Autodesk Inventor part; units mm, degrees
ref_plane "YZ Plane" through (0, 0, 0) normal (1, 0, 0) x (0, 1, 0)
ref_plane "XZ Plane" through (0, 0, 0) normal (0, 1, 0) x (-1, 0, 0)
ref_plane "XY Plane" through (0, 0, 0) normal (0, 0, 1) x (1, 0, 0)
sketch "Original Profile" plane through (0, 0, 0) normal (0, 1, 0) x (-1, 0, 0)
  line L0 (0, 0) -> (-18, 0)
  line L1 (-18, 0) -> (-18, -15)
  line L2 (-18, -15) -> (0, -15)
  line L3 (0, -15) -> (0, 0)
  line L4 (0, -7.5) -> (-18, -7.5)
  circle A0 centre (-11.5, -7.5) radius 1.5
  circle A1 centre (-11.5, -7.5) radius 6.5
  line L5 (-5, -15) -> (-5, 0)
  line L6 (0, -9.0875) -> (-18, -9.0875)
  line L7 (-18, -9.0875) -> (-18, -5.9125)
  line L8 (-18, -5.9125) -> (0, -5.9125)
  line L9 (0, -5.9125) -> (0, -9.0875)
  point P0 (0, -5.9125)
  point P1 (-18, -9.0875)
  dimension "d8" = 3
  dimension "d9" = 13
  dimension "d10" = 15
  dimension "d11" = 11.5
  dimension "d12" = 6.5
  dimension "d15" = 5
  dimension "d32" = 3.175
  dimension "d33" = 3.175
extrude "Stock" add sketch "Original Profile" along normal blind 29.25
sketch "Sketch4" plane through (18, 0, 0) normal (1, 0, 0) x (0, 0, -1)
  line L0 (15, 0) -> (15, 29.25)
  line L1 (0, 21.75) -> (15, 21.75)
  line L2 (15, 21.75) -> (15, 3.75)
  line L3 (15, 3.75) -> (0, 3.75)
  line L4 (0, 3.75) -> (0, 21.75)
  line L5 (0, 0) -> (0, 29.25)
  line L6 (0, 0) -> (15, 0)
  line L7 (15, 29.25) -> (0, 29.25)
  line L8 (7.5, 29.25) -> (7.5, 0) construction
  line L9 (15, 0) -> (0, 0)
  line L10 (2.7375, 0) -> (12.2625, 0)
  line L11 (12.2625, 0) -> (12.2625, 1.5)
  line L12 (12.2625, 1.5) -> (2.7375, 1.5)
  line L13 (2.7375, 1.5) -> (2.7375, 0)
  line L14 (2.7375, 1.5) -> (3.6035, 0)
  line L15 (2.7375, 1.5) -> (4.4696, 1.5) construction
  line L16 (12.2625, 1.5) -> (11.3965, 0)
  line L17 (12.2625, 1.5) -> (13.9946, 1.5) construction
  dimension "d40" = 3.75
  dimension "d41" = 18
  dimension "d44" = 9.525
  dimension "d45" = 4.7625
  dimension "d46" = 1.5
  dimension "d47" = 60
  dimension "d48" = 120
extrude "Cut Slot" cut sketch "Sketch4" against normal blind 14 contours L3 L4 L1 L0
extrude "Extrusion7" cut sketch "Sketch4" against normal through all contours L6 L14 L12 L16
hole "Hole1" at (11.5, 0, -7.5) direction (0, 1, 0) diameter 3.2004 end through all
sketch "Sketch5" plane through (0, 0, 0) normal (-1, 0, 0) x (0, 0, 1)
  circle A0 centre (-7.5, 14.625) radius 1.5
  line L0 (-15, 29.25) -> (0, 29.25)
  line L1 (-15, 0) -> (-11.3965, 0)
  line L2 (-15, 0) -> (-15, 29.25)
  point P0 (0, 0)
  dimension "d51" = 3
  dimension "d52" = 14.625
  dimension "d53" = 29.25
  dimension "d54" = 7.5
hole "Hole2" at (0, 14.625, -7.5) direction (1, 0, 0) diameter 2.459 end through all
chamfer "Chamfer1" distance 7.5 angle 30 1 edges at (18, 25.5, 0) measured on face at (18, 24.25, -10)
chamfer "Chamfer2" distance 7.5 angle 30 1 edges at (18, 1.875, 0) measured on face at (18, 3, -5.9125)
chamfer "Chamfer3" distance 7.5 angle 30 1 edges at (18, 25.5, -15) measured on face at (18, 24.25, -10)
chamfer "Chamfer4" distance 7.5 angle 30 1 edges at (18, 1.875, -15) measured on face at (18, 3, -11.5875)
equation "\"d12\" = 0.5 * d9"
equation "\"d33\" = d32"
equation "\"d45\" = 0.5 * d44"
equation "\"d52\" = 0.5 * d53"
properties part number "Bearing Sled Single" material "Aluminum 6061"
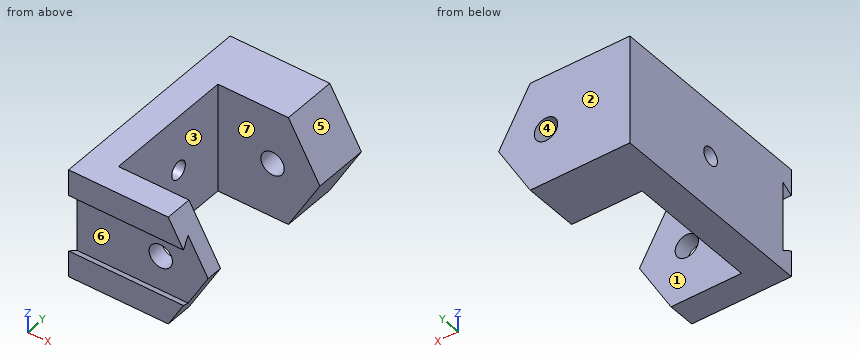
Input: part model. Units: mm. Frame: model coordinates. Face numbers are marked on the shaded views. A direction names the side the tool comes from. Coordinates: 2 decimals unless noted, no trailing zeros. Write each loop counter-clockwise with the first axis right and the second up, starting at its lowest first coordinate (ties: lowest second). Pieces come first, ordered by that corner, then holes. Notation, with made-up numbers: M 79.5,42.25 L 102.5,42.25 A20 cw 102.5,55.25 Z; hole C 78.5,8.5 d8. An arc over 180 degrees is marked long. Answer as a JSON object with one key per item and string values. Group by question number.
(1) Section C-C on x = 6. Output: boundary loops of the cut face in (y, z), plus the area to 3 significant figures.
(2) Ray query, line 1 along Z through (x, y) = (11.5, 24); line 2 along Y through (x, z) = (8.75, -12.5); line 3 along Y through (x, z) = (11.5, -9.5). Return the intervals inside material, ascending. Write a range as [from, to].
(3) Mould query, pull axis Y, two halves, no side actions, for the marked faces 1, 2, 3 and 4. Classes: pulls with the +Y half, pulls with the -Y half, needs draft (parallel to the pull), parting line crosses it, or undercut.
(4) Contact query for flat-ended pins moving along their axis: P1, Ø3.5, axis at x = 11.5, z = -7.5, coming from the -Y side; P2, Ø8, axis at y = 18, z = -11.5, coming from the -X side; P3, Ø4, axis at y = 19.5, z = -13, coming from the +X side. Output: stop coordinate, or through.
(5) Set-up query: the marked faces 5, 6 and 7. Return all of +Z, -Z, +X, -X, +Y, -Y with unobstructed straight access to the full face (end or side cutting, diameter ignored); none if empty.
(6) Section B-B on x = 11.5. Output: boundary loops of the cut face in (y, z), plus the area to 3 significant figures.
(7) Section D-D on z = -4.25. Output: boundary loops of the cut face in (x, y).
Result set:
{
 "1": {"outline": "M 0,-15 L 3.75,-15 L 3.75,0 L 0,0 L 0,-3.6 L 1.5,-2.74 L 1.5,-12.26 L 0,-11.4 Z; M 21.75,-15 L 29.25,-15 L 29.25,0 L 21.75,0 Z", "area": "156 mm2"},
 "2": {"line 1": "z = [-15, -9.1], [-5.9, 0]", "line 2": "y = [0, 3.75], [21.75, 29.25]", "line 3": "y = [1.5, 3.75], [21.75, 29.25]"},
 "3": {"face 1": "undercut", "face 2": "pulls with the +Y half", "face 3": "undercut", "face 4": "needs draft"},
 "4": {"P1": "stops at y = 1.5", "P2": "stops at x = 0", "P3": "stops at x = 4"},
 "5": {"face 5": "+Z, +X, +Y, -Y", "face 6": "+X, -X", "face 7": "+Z, -Z, +X"},
 "6": {"outline": "M 0,-15 L 3.75,-15 L 3.75,-9.1 L 1.5,-9.1 L 1.5,-12.26 L 0,-11.4 Z; M 0,-3.6 L 1.5,-2.74 L 1.5,-5.9 L 3.75,-5.9 L 3.75,0 L 0,0 Z; M 21.75,-15 L 29.25,-15 L 29.25,-9.1 L 21.75,-9.1 Z; M 21.75,-5.9 L 29.25,-5.9 L 29.25,0 L 21.75,0 Z", "area": "125 mm2"},
 "7": {"outline": "M 0,1.5 L 16.12,1.5 L 16.12,3.75 L 4,3.75 L 4,21.75 L 16.12,21.75 L 16.12,29.25 L 0,29.25 Z"}
}
